```python
from build123d import *

# Parameters (mm, degrees)
BOSS_EXTRUDE1_DEPTH = 7.874
SKETCH2_R           = 4.0132
BOSS_EXTRUDE2_DEPTH = 21.3868
SKETCH3_R           = 4.8768
BOSS_EXTRUDE3_DEPTH = 52.6288
SKETCH10_W          = 30.48
SKETCH10_H          = 3.81
FILLET1_R           = 1.27
FILLET2_R           = 1.27


with BuildPart() as part:
    # Sketch1 → Boss-Extrude1 (new body)
    with BuildSketch(Plane.XY):
        Polygon((4.8552834, 2.881406504), (-0.067729531, 5.645502019), (-4.923012931, 2.764095515), (-4.8552834, -2.881406504), (0.067729531, -5.645502019), (4.923012931, -2.764095515), align=None)
    extrude(amount=BOSS_EXTRUDE1_DEPTH)

    # Sketch2 → Boss-Extrude2 (add)
    with BuildSketch(Plane.XY.offset(7.874)):
        with Locations(Location((0, 0, 0), (0, 0, 180))):
            Circle(SKETCH2_R)
    extrude(amount=BOSS_EXTRUDE2_DEPTH)

    # Sketch3 → Boss-Extrude3 (add)
    with BuildSketch(Plane(origin=(0, 0, 0), x_dir=(-1, 0, 0), z_dir=(0, 0, -1))):
        Circle(SKETCH3_R)
    extrude(amount=BOSS_EXTRUDE3_DEPTH)

    # Sketch8 → Cut-Revolve1 (revolve, cut)
    with BuildSketch(Plane(origin=(0, 0, 0), x_dir=(0, 0, -1), z_dir=(1, 0, 0)), mode=Mode.PRIVATE) as cut_revolve1_sk:
        Polygon((0, 3.9116), (2.54, 3.9116), (4.896343106, 6.267943106), (4.896343106, 7.7216), (0, 7.7216), align=None)
    revolve(cut_revolve1_sk.sketch.rotate(Axis((0, 0, -56.72328), (0, 0, 1)), 90), axis=Axis((0, 0, -56.72328), (0, 0, 1)), mode=Mode.SUBTRACT)

    # Sketch9 → Cut-Revolve2 (revolve, cut)
    with BuildSketch(Plane(origin=(0, 0, 0), x_dir=(0, 0, -1), z_dir=(1, 0, 0)), mode=Mode.PRIVATE) as cut_revolve2_sk:
        Polygon((16.6878, 3.9116), (14.870743755, 5.728656245), (14.870743755, 7.7216), (25.5778, 7.7216), (25.5778, 3.9116), align=None)
    revolve(cut_revolve2_sk.sketch.rotate(Axis((0, 0, -56.72328), (0, 0, 1)), 270), axis=Axis((0, 0, -56.72328), (0, 0, 1)), mode=Mode.SUBTRACT)

    # Sketch10 → Cut-Revolve3 (revolve, cut)
    with BuildSketch(Plane(origin=(0, 0, 0), x_dir=(0, 0, -1), z_dir=(1, 0, 0)), mode=Mode.PRIVATE) as cut_revolve3_sk:
        with Locations((40.8178, 4.4196)):
            Rectangle(SKETCH10_W, SKETCH10_H)
    revolve(cut_revolve3_sk.sketch.rotate(Axis((0, 0, -56.72328), (0, 0, 1)), 270), axis=Axis((0, 0, -56.72328), (0, 0, 1)), mode=Mode.SUBTRACT)

    # Fillet1
    fillet1_edges = [part.edges().sort_by_distance(p)[0] for p in [
        (-2.5146, 0, -52.6288),
    ]]
    fillet(fillet1_edges, radius=FILLET1_R)

    # Sketch13 → Cut-Revolve4 (revolve, cut)
    with BuildSketch(Plane(origin=(0, 0, 0), x_dir=(0, 0, -1), z_dir=(1, 0, 0)), mode=Mode.PRIVATE) as cut_revolve4_sk:
        Polygon((-10.033, 4.0132), (-11.3919, 2.6543), (-14.9479, 2.6543), (-15.691743647, 3.398143647), (-20.898743647, 3.398143647), (-20.898743647, 1.9812), (-29.2608, 1.9812), (-29.2608, 6.514945502), (-10.033, 6.514945502), align=None)
    revolve(cut_revolve4_sk.sketch.rotate(Axis((0, 0, -56.72328), (0, 0, 1)), 90), axis=Axis((0, 0, -56.72328), (0, 0, 1)), mode=Mode.SUBTRACT)

    # Fillet2
    fillet2_edges = [part.edges().sort_by_distance(p)[0] for p in [
        (1.9812, 0, 29.2608),
    ]]
    fillet(fillet2_edges, radius=FILLET2_R)


solid = part.part
```
Can you work these out from the model? Positions are in its coordinate system, mm. A direction names the side the tool comes from. Give positions to 0.01 mm unless a question says otherwise; leave off trailing zeros. Write each loop counter-clockwise with the first axis right and the second up, starting at its lowest first coordinate (ties: lowest second). Pieces come first, ordered by that corner, then holes. Notation, with made-up numbers: (45, 44) -> (90, 44) arc R20 ccw to (90, 48) -> close; hole circle Ø2 at (54, 49.5). An arc over 180 degrees is marked (long way). One line per item, written item: value.
Q1. Imagine slicing it at B-B on z = 17. Please give me the cut outline in (x, y).
Results found:
outline: circle Ø6.8 at (0, 0)
Q2. Which directions (+Z, -Z, +X, -X, +Y, -Y) give clear straight access to the entire face, cutting with the end or side of a thin tool? Please do faces 1 (the face through (-1.996, -1.53, -38.649)), 2 (the face through (-2.428, -4.244, 3.882)), 3 (the face through (2.96, -2.71, 8.94)).
Results found:
face 1: -Z
face 2: +Z, -Z, -X, -Y
face 3: +Z
Q3. We'd pull the mould along Z, two halves only. Please class faces 4 (the face through (0, -3, -25.578)), 5 (the face through (0, 2.2, 20.899)), 6 (the face through (0.35, -2.63, 13.19)): +Z half, -Z half, draft (parallel to the pull), parting line (faces both ways), or undercut.
Results found:
face 4: -Z half
face 5: +Z half
face 6: undercut
Q4. Imagine slicing it at A-A on z = -20. Please give me the cut outline in (x, y).
Results found:
outline: circle Ø7.82 at (0, 0)
Q5. For P1, Ø1.5, axis at x = 0.5, y = -2, coming from the +Z side; P2, Ø5, axis at x = 0.5, z = -15.5, coming from the -Y side; P3, Ø3, axis at y = 2.5, z = -43, coming from the +X side, each with a flat end and sliding along its axis, tell me the tip position at first contact or that it passes through.
Results found:
P1: stops at z = 29.11
P2: stops at y = -4.88
P3: stops at x = 2.31
Q6. Please list where these lines run through material, in increasing order: line 1 (Y direction, x = 3, z = 5); line 2 (Y direction, x = -3, z = 10); line 3 (X direction, y = 2.75, z = 19). Write a range as [from, to].
Results found:
line 1: y = [-3.91, 3.92]
line 2: y = [-2.67, 2.67]
line 3: x = [-2, 2]
